Can you work these out from the model? Positions are in its coordinate system, mm. A direction names the side the tool comes from. Coordinates: 2 decimals unless noted, no trailing zeros. Order: outer loops, then holes, each group sorted by start corner. A loop starts at its lowest first (then second) coordinate and runs counter-clockwise, first axis right, second up.
```python
from build123d import *

# Parameters (mm, degrees)
F0_R     = 11.6
F0_R_2   = 9.6
F1_DEPTH = 5.2
F2_R     = 11.6
F2_R_2   = 9.6
F3_DEPTH = 2
F4_W     = 40
F4_H     = 30
F4_R     = 11.6
F5_DEPTH = 7.2
F6_R     = 5
F7_R     = 10.8681902922
F7_R_2   = 9.8681902922
F7_W     = 3.8435366005
F7_H     = 6.8932622671
F7_R_3   = 2.0674977133
F8_DEPTH = 2


with BuildPart() as f1:
    # F0 (on Top) → F1 (new body)
    with BuildSketch(Plane.XY):
        Circle(F0_R)
        Circle(F0_R_2, mode=Mode.SUBTRACT)
    extrude(amount=F1_DEPTH)

    # F2 (on face) → F3 (join)
    with BuildSketch(Plane.XY.offset(5.2)):
        Circle(F2_R)
        Circle(F2_R_2, mode=Mode.SUBTRACT)
        Circle(F2_R_2)
    extrude(amount=F3_DEPTH)

    # F4 (on face) → F5 (join)
    with BuildSketch(Plane.XY.offset(7.2)):
        Rectangle(F4_W, F4_H)
        Circle(F4_R, mode=Mode.SUBTRACT)
    extrude(amount=-F5_DEPTH)

    # F6
    f6_edges = [f1.edges().sort_by_distance(p)[0] for p in [
        (-20, -15, 3.6),
        (-20, 15, 3.6),
        (20, -15, 3.6),
        (20, 15, 3.6),
    ]]
    fillet(f6_edges, radius=F6_R)

    # F7 (on face) → F8 (join)
    with BuildSketch(Plane.XY.offset(7.2)):
        with Locations((6.3613462262, 0)):
            Circle(F7_R)
        with Locations((6.3613462262, 0)):
            Circle(F7_R_2, mode=Mode.SUBTRACT)
        with BuildLine():
            ThreePointArc((1.6207129094, 4.9697518697), (3.6583417714, -6.3139373459), (13.2295365184, 0))
            ThreePointArc((13.2295365184, 0), (12.6752835721, 2.7030044548), (11.1019795429, 4.9697518697))
            Line((11.1019795429, 4.9697518697), (1.6207129094, 4.9697518697))
        make_face()
        with Locations((-14.2829688266, -8.0176712945)):
            Rectangle(F7_W, F7_H)
        with Locations((-14.2829688266, 7.2108898312)):
            Circle(F7_R_3)
        with Locations((-14.2829688266, 12.2118974105)):
            Circle(F7_R_3)
    extrude(amount=F8_DEPTH)


solid = f1.part
```
1. Imagine slicing it at D-D on x = -7.5. Please give me the cut outline in (y, z), then the cut area to 3 significant figures.
Completed:
outline: (-15, 0) - (-5.99, 0) - (-5.99, 5.2) - (5.99, 5.2) - (5.99, 0) - (15, 0) - (15, 7.2) - (-15, 7.2) - close
area: 154 mm2
2. Thinking about a two-plate mould opening in Y: for faces 5 (the cylindrical face through (18, -14, 4)), 6 (the flat face through (6, 4.97, 8)), 7 (the flat face through (0, 15, 4)), which applies, pulls with the +Y half, pulls with the -Y half, needs draft (parallel to the pull), parting line crosses it, or undercut?
Completed:
face 5: pulls with the -Y half
face 6: undercut
face 7: pulls with the +Y half
3. I'm going to push flat-ended pins straight in: pin 1 (1 mm diameter, centred on y = -7, z = 8, fed in from -X); pin 2 (2 mm diameter, centred on x = -15, z = 8.5, fed in from -Y); pin 3 (3 mm diameter, centred on x = -6.5, y = 2.5, fed in from +Z). Where does each tip first touch, or does it pass through?
Completed:
pin 1: stops at x = -16.2
pin 2: stops at y = -11.46
pin 3: stops at z = 7.2
4. Imagine slicing it at B-B on x = 12. Please give me the cut outline in (y, z), then the cut area to 3 significant figures.
Completed:
outline: (-15, 0) - (15, 0) - (15, 7.2) - (9.29, 7.2) - (9.29, 9.2) - (8.1, 9.2) - (8.1, 7.2) - (3.92, 7.2) - (3.92, 9.2) - (-3.92, 9.2) - (-3.92, 7.2) - (-8.1, 7.2) - (-8.1, 9.2) - (-9.29, 9.2) - (-9.29, 7.2) - (-15, 7.2) - close
area: 236 mm2
5. Imagine slicing it at C-C on y = -2. Please give me the cut outline in (x, z), then the cut area to 3 significant figures.
Completed:
outline: (-20, 0) - (-9.39, 0) - (-9.39, 5.2) - (9.39, 5.2) - (9.39, 0) - (20, 0) - (20, 7.2) - (17.04, 7.2) - (17.04, 9.2) - (16.02, 9.2) - (16.02, 7.2) - (12.93, 7.2) - (12.93, 9.2) - (-0.21, 9.2) - (-0.21, 7.2) - (-3.3, 7.2) - (-3.3, 9.2) - (-4.32, 9.2) - (-4.32, 7.2) - (-20, 7.2) - close
area: 221 mm2
6. Imagine slicing it at A-A on z = 4.75. Please give me the cut outline in (x, y), then the cut area to 3 significant figures.
Completed:
outline: (-20, -10) arc R5 ccw to (-15, -15) - (15, -15) arc R5 ccw to (20, -10) - (20, 10) arc R5 ccw to (15, 15) - (-15, 15) arc R5 ccw to (-20, 10) - close; hole circle Ø19.2 at (0, 0)
area: 889 mm2
7. Please list where these lines run through material, in increasing order: probe 1 along Y at (x, z) = (0, 2.6); probe 2 along X at (y, z) = (5.75, 7.25); probe 3 along Y at (x, z) = (8.5, 7.25).
Completed:
probe 1: y = -15 to -9.6, 9.6 to 15
probe 2: x = -15.75 to -12.82, -2.86 to -1.66, 14.38 to 15.58
probe 3: y = -10.66 to -9.63, -6.53 to 4.97, 9.63 to 10.66
8. On a 3-axis mill with a long thin cutter (end or side, diameter ignored), from which of +Z, -Z, +X, -X, +Y, -Y can I reach the whole of each face in a straight line? I mean faces 1 (the flat face through (-14, -4.571, 8)), 2 (the flat face through (-12.361, -8, 8)), 3 (the flat face through (6, 7, 7.2)), 4 (the cylindrical face through (5.161, 8.095, 2.564)). Say none if no direction works.
Completed:
face 1: +Z, -X
face 2: +Z, -Y
face 3: +Z
face 4: -Z
